from build123d import *

# Parameters (mm, degrees)
F0_W     = 141.2875
F0_H     = 255.393249
F0_R     = 6.746875
F0_R_2   = 64.29375
F0_R_3   = 4.7625
F1_DEPTH = 6.35
F2_R     = 12.7


with BuildPart() as f1:
    # F0 (on Front) → F1 (new body)
    with BuildSketch(Plane.XZ):
        with Locations((-57.94375, -114.996624)):
            Rectangle(F0_W, F0_H)
        with Locations((-109.343249, -217.293249)):
            Circle(F0_R, mode=Mode.SUBTRACT)
        with Locations((-4.956751, -217.293249)):
            Circle(F0_R, mode=Mode.SUBTRACT)
        with Locations((-57.15, -165.1)):
            Circle(F0_R_2, mode=Mode.SUBTRACT)
        with Locations((-109.343249, -112.906751)):
            Circle(F0_R, mode=Mode.SUBTRACT)
        with Locations((-95.25, -50.8)):
            Circle(F0_R_3, mode=Mode.SUBTRACT)
        with Locations((-115.8875, 0)):
            Circle(F0_R_3, mode=Mode.SUBTRACT)
        with Locations((-4.956751, -112.906751)):
            Circle(F0_R, mode=Mode.SUBTRACT)
        with Locations((0, -50.8)):
            Circle(F0_R_3, mode=Mode.SUBTRACT)
        Circle(F0_R_3, mode=Mode.SUBTRACT)
    extrude(amount=F1_DEPTH)

    # F2
    f2_edges = [f1.edges().sort_by_distance(p)[0] for p in [
        (-128.5875, -3.175, -242.693249),
        (12.7, -3.175, -242.693249),
        (12.7, -3.175, 12.7),
        (-128.5875, -3.175, 12.7),
    ]]
    fillet(f2_edges, radius=F2_R)


solid = f1.part
Verification items for the finished model (mm, model axes). Give positions to 0.01 mm unless a question says otherwise; leave off trailing zeros. Loops run counter-clockwise (first coordinate to the right, second up) from the corner with the lowest first, then second, coordinate; pieces in that order, holes last.
1) Sectioned sample at C-C, the plane z = -165.1. Enter the section's corners in (x, y).
2) Depth check by flat-ended pin: pin 1 Ø8 at (x, z) = (-107, -201.5) entering from +Y; pin 2 Ø11 at (x, z) = (-109.34, -217.29) entering from +Y. Enter the tip coordinate at first touch or a pass-through.
3) Sectioned sample at B-B, the plane z = -50.8. Enter the section's corners in (x, y), then the cut area to 3 significant figures.
4) Thickness scan on line 1 along Z through (x, y) = (-114.5, -5.25); line 2 along Z through (x, y) = (-99, -5.25); line 3 along Z through (x, y) = (0, -2.5). Record the ranges inside material, lowest first.
5) Draft check along Z on faces 1 (the cylindrical face through (8.88, -3.22, -239.07)), 2 (the cylindrical face through (-3.78, -3.13, -2.9)), 3 (the flat face through (12.7, -3, -117)), 4 (the cylindrical face through (-124.966, -3.219, 8.881)). Enter one of: pulls with the +Z half, pulls with the -Z half, needs draft (parallel to the pull), parting line crosses it, or undercut.
6) Sectioned sample at A-A, the plane x = -57.15. Enter the section's corners in (y, z), then the cut area to 3 significant figures.
7) Sectioned sample at D-D, the plane y = -4. Count the separate pieces of the cut face and the enclosed holes in it, then the cut area to 3 significant figures.
Answers:
1. outline: (-128.59, -6.35) - (-121.44, -6.35) - (-121.44, 0) - (-128.59, 0) - close; (7.14, -6.35) - (12.7, -6.35) - (12.7, 0) - (7.14, 0) - close
2. pin 1: stops at y = 0
2. pin 2: passes through
3. outline: (-128.59, -6.35) - (-100.01, -6.35) - (-100.01, 0) - (-128.59, 0) - close; (-90.49, -6.35) - (-4.76, -6.35) - (-4.76, 0) - (-90.49, 0) - close; (4.76, -6.35) - (12.7, -6.35) - (12.7, 0) - (4.76, 0) - close
3. area: 776 mm2
4. line 1: z = -242.69 to -221.64, -212.94 to -194.16, -136.04 to -117.26, -108.56 to -4.56, 4.56 to 12.7
4. line 2: z = -242.69 to -213.91, -116.29 to -53.74, -47.86 to 12.7
4. line 3: z = -242.69 to -221.87, -212.72 to -194.55, -135.65 to -117.48, -108.33 to -55.56, -46.04 to -4.76, 4.76 to 12.7
5. face 1: pulls with the -Z half
5. face 2: undercut
5. face 3: needs draft
5. face 4: pulls with the +Z half
6. outline: (-6.35, -242.69) - (0, -242.69) - (0, -229.39) - (-6.35, -229.39) - close; (-6.35, -100.81) - (0, -100.81) - (0, 12.7) - (-6.35, 12.7) - close
6. area: 805 mm2
7. separate pieces: 1
7. enclosed holes: 9
7. area: 22,100 mm2
